```python
from build123d import *
from build123d.topology import SkipClean

# Parameters (mm, degrees)
CUT_EXTRUDE1_START       = -11.734260502
CUT_EXTRUDE1_OUTLINE_R   = 34.671
CUT_EXTRUDE1_DEPTH       = 11.182953842
CUT_EXTRUDE1_START_2     = -0.55130666
CUT_EXTRUDE1_2_OUTLINE_R = 24.1554
CUT_EXTRUDE1_2_DEPTH     = 0.856646158
CUT_EXTRUDE1_3_DEPTH     = 0.55130666
CUT_EXTRUDE1_START_3     = -0.79375
CUT_EXTRUDE1_5_DEPTH     = 1.5875
CUT_EXTRUDE2_START       = -0.55130666
CUT_EXTRUDE2_DEPTH       = 0.55130666
BOSS_EXTRUDE1_DEPTH      = 0.55130666
BOSS_EXTRUDE2_DEPTH      = 0.55130666
BOSS_EXTRUDE3_DEPTH      = 0.965739498
BOSS_EXTRUDE4_DEPTH      = 0.965739498
SKETCH7_R                = 20.955
CUT_EXTRUDE3_DEPTH       = 0.6096
M6_CLEARANCE_HOLE1_D     = 6.731
M6_CLEARANCE_HOLE2_D     = 6.731
CHAMFER1_SIZE            = 0.381
CHAMFER2_SIZE            = 0.762


with BuildPart() as part:
    # Cut-Extrude1: read off the stored shape, not the designer's step
    # Cut-Extrude1 outline → Cut-Extrude1 (new body)
    with BuildSketch(Plane.XY.offset(-0.965739498).offset(CUT_EXTRUDE1_START)):
        Circle(CUT_EXTRUDE1_OUTLINE_R)
    extrude(amount=CUT_EXTRUDE1_DEPTH)

    # Cut-Extrude1 2 outline → Cut-Extrude1 2 (add)
    with BuildSketch(Plane.XY.offset(-0.965739498).offset(CUT_EXTRUDE1_START_2)):
        Circle(CUT_EXTRUDE1_2_OUTLINE_R)
    extrude(amount=CUT_EXTRUDE1_2_DEPTH)

    # Cut-Extrude1 3 outline → Cut-Extrude1 3 (add)
    with BuildSketch(Plane.XY.offset(-0.965739498).offset(CUT_EXTRUDE1_START_2)):
        with BuildLine():
            Line((12.758585218, 20.51101783), (18.018364086, 29.621222066))
            ThreePointArc((18.018364086, 29.621222066), (-30.025966775, 17.3355), (-16.643548757, -30.414972066))
            Line((-16.643548757, -30.414972066), (-11.383769889, -21.30476783))
            ThreePointArc((-11.383769889, -21.30476783), (-20.919190039, 12.0777), (12.758585218, 20.51101783))
        make_face()
    extrude(amount=CUT_EXTRUDE1_3_DEPTH)

    # Cut-Extrude1 4 outline → Cut-Extrude1 4 (revolve, cut)
    with BuildSketch(Plane.XZ):
        Polygon((24.1554, -1.825250338), (24.1554, -0.6604), (20.955, -0.6604), align=None)
    revolve(axis=Axis((0, 0, 0), (0, 0, 1)), mode=Mode.SUBTRACT)

    # Cut-Extrude1 5 outline → Cut-Extrude1 5 (cut)
    with BuildSketch(Plane(origin=(0, 0, 0), x_dir=(0.49999999999977696, 0.8660254037845674, 0), z_dir=(0.8660254037845674, -0.4999999999997772, 0)).offset(CUT_EXTRUDE1_START_3)):
        Polygon((36, -0.965739498), (24.142355107, -0.965739498), (34.671, -1.517522396), (36, -1.587172335), align=None)
        Polygon((-34.671, -1.517522396), (-24.142355107, -0.965739498), (-36, -0.965739498), (-36, -1.587172335), align=None)
    extrude(amount=CUT_EXTRUDE1_5_DEPTH, mode=Mode.SUBTRACT)

    # Sketch2 → Cut-Extrude2 (cut)
    with BuildSketch(Plane.XY.offset(-0.965739498).offset(CUT_EXTRUDE2_START)):
        with BuildLine():
            Line((-18.018364086, -29.621222066), (-12.758585218, -20.51101783))
            ThreePointArc((-12.758585218, -20.51101783), (-20.919190039, 12.0777), (11.383769889, 21.30476783))
            Line((11.383769889, 21.30476783), (16.643548757, 30.414972066))
            ThreePointArc((16.643548757, 30.414972066), (-30.025966775, 17.3355), (-18.018364086, -29.621222066))
        make_face()
    extrude(amount=CUT_EXTRUDE2_DEPTH, mode=Mode.SUBTRACT)

    # Sketch3 → Boss-Extrude1 (add)
    with SkipClean():  # the faces are left unmerged after this step: merging them gives an invalid solid
        with BuildSketch(Plane.XY.offset(-1.517046158)):
            with BuildLine():
                Line((-16.643548757, -30.414972066), (-11.383769889, -21.30476783))
                ThreePointArc((-11.383769889, -21.30476783), (20.919190039, -12.0777), (12.758585218, 20.51101783))
                Line((12.758585218, 20.51101783), (18.018364086, 29.621222066))
                ThreePointArc((18.018364086, 29.621222066), (30.025966775, -17.3355), (-16.643548757, -30.414972066))
            make_face()
        extrude(amount=BOSS_EXTRUDE1_DEPTH)

    # Sketch4 → Boss-Extrude2 (add)
    with SkipClean():  # the faces are left unmerged after this step: merging them gives an invalid solid
        with BuildSketch(Plane.XY.offset(-1.517046158)):
            with BuildLine():
                Line((16.643548757, 30.414972066), (11.383769889, 21.30476783))
                ThreePointArc((11.383769889, 21.30476783), (-20.919190039, 12.0777), (-12.758585218, -20.51101783))
                Line((-12.758585218, -20.51101783), (-18.018364086, -29.621222066))
                ThreePointArc((-18.018364086, -29.621222066), (-30.025966775, 17.3355), (16.643548757, 30.414972066))
            make_face()
        extrude(amount=BOSS_EXTRUDE2_DEPTH)

    # Sketch5 → Boss-Extrude3 (add)
    with SkipClean():  # the faces are left unmerged after this step: merging them gives an invalid solid
        with BuildSketch(Plane.XY.offset(-0.965739498)):
            with BuildLine():
                Line((-16.643548757, -30.414972066), (-11.383769889, -21.30476783))
                ThreePointArc((-11.383769889, -21.30476783), (20.919190039, -12.0777), (12.758585218, 20.51101783))
                Line((12.758585218, 20.51101783), (18.018364086, 29.621222066))
                ThreePointArc((18.018364086, 29.621222066), (30.025966775, -17.3355), (-16.643548757, -30.414972066))
            make_face()
        extrude(amount=BOSS_EXTRUDE3_DEPTH)

    # Sketch6 → Boss-Extrude4 (add)
    with SkipClean():  # the faces are left unmerged after this step: merging them gives an invalid solid
        with BuildSketch(Plane.XY.offset(-0.965739498)):
            with BuildLine():
                Line((16.643548757, 30.414972066), (11.383769889, 21.30476783))
                ThreePointArc((11.383769889, 21.30476783), (-20.919190039, 12.0777), (-12.758585218, -20.51101783))
                Line((-12.758585218, -20.51101783), (-18.018364086, -29.621222066))
                ThreePointArc((-18.018364086, -29.621222066), (-30.025966775, 17.3355), (16.643548757, 30.414972066))
            make_face()
        extrude(amount=BOSS_EXTRUDE4_DEPTH)

    # Sketch7 → Cut-Extrude3 (cut)
    with SkipClean():  # the faces are left unmerged after this step: merging them gives an invalid solid
        with BuildSketch(Plane.XY.offset(-0.6604)):
            with Locations(Location((0, 0, 0), (0, 0, 180))):
                Circle(SKETCH7_R)
        extrude(amount=-CUT_EXTRUDE3_DEPTH, mode=Mode.SUBTRACT)

    # M6 Clearance Hole1 (through all)
    with Locations(Plane(origin=(0, 0, -12.7), x_dir=(-1, 0, 0), z_dir=(0, 0, -1))):
        with Locations((-25.428584316, 14.6812)):
            Hole(M6_CLEARANCE_HOLE1_D / 2)

    # M6 Clearance Hole2 (through all)
    with Locations(Plane.XY):
        with Locations((0, 29.3624), (25.428584316, -14.6812), (0, -29.3624), (-25.428584316, -14.6812), (-25.428584316, 14.6812)):
            Hole(M6_CLEARANCE_HOLE2_D / 2)

    # Chamfer1
    chamfer1_edges = [part.edges().sort_by_distance(p)[0] for p in [
        (22.063084316, 14.6812, -12.7),
        (22.063084316, 14.6812, 0),
        (-22.063084316, 14.6812, 0),
        (-22.063084316, 14.6812, -12.7),
        (-22.063084316, -14.6812, 0),
        (-22.063084316, -14.6812, -12.7),
        (3.3655, -29.3624, 0),
        (3.3655, -29.3624, -12.7),
        (28.794084316, -14.6812, 0),
        (28.794084316, -14.6812, -12.7),
        (3.3655, 29.3624, 0),
        (3.3655, 29.3624, -12.7),
    ]]
    chamfer(chamfer1_edges, length=CHAMFER1_SIZE)

    # Chamfer2
    chamfer2_edges = [part.edges().sort_by_distance(p)[0] for p in [
        (30.025966775, -17.3355, 0),
        (-30.025966775, 17.3355, 0),
        (-34.671, 0, -12.7),
    ]]
    chamfer(chamfer2_edges, length=CHAMFER2_SIZE)


solid = part.part
```
Here's how the part is built. I have some questions about the finished solid (model axes, mm). A direction names the side the tool comes from. Round coordinates to 2 decimals unless told otherwise and drop trailing zeros. Order: outer loops, then holes, each group sorted by start corner. A loop starts at its lowest first (then second) coordinate and runs counter-clockwise, first axis right, second up. Notation, with made-up numbers: M 4.5,-32.5 L 21.5,-32.5 A20 ccw 21.5,-12.5 Z; hole C 8.5,14.5 d7. An arc over 180 degrees is marked long. One line per question, with ' | ' between items.
1) I want a section at B-B, the plane y = 0. Write out the boundary of the cut face in (x, z) (3 decimals), then the cut area to 3 significant figures.
Working result:
outline: M -34.671,-11.938 L -33.909,-12.7 L 33.909,-12.7 L 34.671,-11.938 L 34.671,-0.762 L 33.909,0 L 24.155,0 L 24.155,-1.825 L 20.955,-0.66 L 20.955,-1.27 L -20.955,-1.27 L -20.955,-0.66 L -24.155,-1.825 L -24.155,0 L -33.909,0 L -34.671,-0.762 Z | area: 818 mm²
2) For pin 1 Ø11 at (x, y) = (0, 29.36) entering from -Z; pin 2 Ø1.5 at (y, z) = (25, -1.5) entering from -X; pin 3 Ø3 at (x, z) = (20, -6) entering from +Y; pin 4 Ø5 at (x, z) = (19.5, -8.5) entering from +Y, each with a flat end and sliding along its axis, tell me the tip position at first contact or that it passes through.
Working result:
pin 1: z = -12.7 | pin 2: x = -24.78 | pin 3: y = 29.32 | pin 4: y = 30.22
3) I want a section at C-C, the plane z = -10.25. Write out the boundary of the cut face in (x, y).
Working result:
outline: C 0,0 d69.34; hole C -25.43,-14.68 d6.73; hole C -25.43,14.68 d6.73; hole C 0,-29.36 d6.73; hole C 0,29.36 d6.73; hole C 25.43,-14.68 d6.73; hole C 25.43,14.68 d6.73
4) For faces 1 (the face through (0, 0, -12.7)), 2 (the face through (2.728, -20.777, -0.961)), which set-ups out of +Z, -Z, +X, -X, +Y, -Y let a thin tool reach every point of the face, with its end or its side?
Working result:
face 1: -Z, +X, -X, +Y, -Y | face 2: +Z
5) I need wall thicknesses on line 1 along Y through (x, z) = (0, -4.25); line 2 along X through (y, z) = (-15.5, -11); line 3 along Y through (x, z) = (2.5, -10). Which ranges of each line are inside material? Lowest first, please.
Working result:
line 1: -34.67 to -32.73, -26 to 26, 32.73 to 34.67 | line 2: -31.01 to -28.69, -22.16 to 22.16, 28.69 to 31.01 | line 3: -34.58 to -31.62, -27.11 to 27.11, 31.62 to 34.58
6) I want a section at A-A, the plane x = 0. State how many separate pieces and enclosed holes the cut face has, then the cut area to 3 significant figures.
Working result:
separate pieces: 3 | enclosed holes: 0 | area: 647 mm²
7) If we mould it in two halves opening along Y, with no side actions, what happens to faces 3 (the face through (-22, 12, 0)), 4 (the face through (-22.95, 16.96, -6.43)), 5 (the face through (0, 0, -1.27))? For each: +Y half, -Y half, draft (parallel to the pull), parting line (faces both ways), or undercut.
Working result:
face 3: draft | face 4: undercut | face 5: undercut
